```python
from build123d import *

# Parameters (mm, degrees)
F0_W         = 22.86
F0_H         = 48.26
F1_DEPTH     = 50.8
F2_W         = 15.24
F2_H         = 6.35
F3_DEPTH     = 41.91
F4_T1_DEPTH  = 3.81
F4_T3_DEPTH  = 3.81
F4_T8_DEPTH  = 56.8427535009
F4_T14_DEPTH = 56.8427535009
F4_T20_DEPTH = 56.8427535009
F4_T26_DEPTH = 56.8427535009
F5_R         = 7.61999
F6_DEPTH     = 2.54
F7_R         = 3.81
F8_R         = 2.54
F9_DEPTH     = 25.4


# Not quite as in the source:
# - a fillet or chamfer that OpenCascade refuses, or shapes differently, is made with other operations: its cross-section is extruded or revolved along the edge and cut away or added
# - a fillet or chamfer is up to 0.001 mm smaller than in the source, because OpenCascade refuses the exact size


with BuildPart() as f1:
    # F0 (on Top) → F1 (new body)
    with BuildSketch(Plane.XY):
        Rectangle(F0_W, F0_H)
    extrude(amount=F1_DEPTH)

    # F2 (on face) → F3 (cut)
    with BuildSketch(Plane.XY.offset(50.8)):
        Polygon((11.43, 24.13), (-11.43, 24.13), (-11.43, 12.7), (-7.62, 12.7), (7.62, 12.7), (11.43, 12.7), align=None)
        with Locations((0, 9.525)):
            Rectangle(F2_W, F2_H)
        Polygon((-11.43, -12.7), (-11.43, -24.13), (11.43, -24.13), (11.43, -12.7), (7.62, -12.7), (-7.62, -12.7), align=None)
        with Locations((0, -9.525)):
            Rectangle(F2_W, F2_H)
    extrude(amount=-F3_DEPTH, mode=Mode.SUBTRACT)

    # F4: fillet of radius 25.4 on 4 edges, made by hand

    # F4_s2 → F4_t1 (join)
    with BuildSketch(Plane.YZ.offset(-11.43)):
        with BuildLine():
            ThreePointArc((-24.1299175004, 8.889874725), (-15.7392117545, 18.0547879388), (-12.69985, 30.1031013998))
            Line((-12.69985, 30.1031013998), (-12.19185, 30.1031013998))
            ThreePointArc((-12.19185, 30.1031013998), (-12.192, 19.4965506999), (-12.192, 8.89))
            Line((-12.192, 8.89), (-12.7, 8.382))
            ThreePointArc((-12.7, 8.382), (-18.4149587502, 8.382), (-23.8505188504, 8.4656101915))
            Line((-23.8505188504, 8.4656101915), (-24.1299175004, 8.889874725))
        make_face()
        with BuildLine():
            ThreePointArc((24.1299175004, 8.889874725), (15.7392117545, 18.0547879388), (12.69985, 30.1031013998))
            Line((12.69985, 30.1031013998), (12.19185, 30.1031013998))
            ThreePointArc((12.19185, 30.1031013998), (12.192, 19.4965506999), (12.192, 8.89))
            Line((12.192, 8.89), (12.7, 8.382))
            ThreePointArc((12.7, 8.382), (18.4149587502, 8.382), (23.8505188504, 8.4656101915))
            Line((23.8505188504, 8.4656101915), (24.1299175004, 8.889874725))
        make_face()
    extrude(amount=F4_T1_DEPTH)

    # F4_s4 → F4_t3 (join)
    with BuildSketch(Plane.YZ.offset(7.62)):
        with BuildLine():
            ThreePointArc((-24.1299175004, 8.889874725), (-15.7392117545, 18.0547879388), (-12.69985, 30.1031013998))
            Line((-12.69985, 30.1031013998), (-12.19185, 30.1031013998))
            ThreePointArc((-12.19185, 30.1031013998), (-12.192, 19.4965506999), (-12.192, 8.89))
            Line((-12.192, 8.89), (-12.7, 8.382))
            ThreePointArc((-12.7, 8.382), (-18.4149587502, 8.382), (-23.8505188504, 8.4656101915))
            Line((-23.8505188504, 8.4656101915), (-24.1299175004, 8.889874725))
        make_face()
        with BuildLine():
            ThreePointArc((24.1299175004, 8.889874725), (15.7392117545, 18.0547879388), (12.69985, 30.1031013998))
            Line((12.69985, 30.1031013998), (12.19185, 30.1031013998))
            ThreePointArc((12.19185, 30.1031013998), (12.192, 19.4965506999), (12.192, 8.89))
            Line((12.192, 8.89), (12.7, 8.382))
            ThreePointArc((12.7, 8.382), (18.4149587502, 8.382), (23.8505188504, 8.4656101915))
            Line((23.8505188504, 8.4656101915), (24.1299175004, 8.889874725))
        make_face()
    extrude(amount=F4_T3_DEPTH)


with BuildPart() as f4_tool6:
    # F4_s7 → F4_t8 (new body)
    with BuildSketch(Plane.YZ.offset(45.4127535009)):
        with BuildLine():
            ThreePointArc((-24.1299175004, 8.889874725), (-15.7392117545, 18.0547879388), (-12.69985, 30.1031013998))
            Line((-12.69985, 30.1031013998), (-12.19185, 30.1031013998))
            ThreePointArc((-12.19185, 30.1031013998), (-12.192, 19.4965506999), (-12.192, 8.89))
            Line((-12.192, 8.89), (-12.7, 8.382))
            ThreePointArc((-12.7, 8.382), (-18.4149587502, 8.382), (-23.8505188504, 8.4656101915))
            Line((-23.8505188504, 8.4656101915), (-24.1299175004, 8.889874725))
        make_face()
    extrude(amount=-F4_T8_DEPTH)

    split(bisect_by=Plane.YZ.offset(11.43), keep=Keep.BOTTOM)

    split(bisect_by=Plane.YZ.offset(7.62), keep=Keep.TOP)


with BuildPart() as f1_1:
    add(f1.part)

    # F4_t5: union F4_tool6
    add(f4_tool6.part)


with BuildPart() as f4_tool12:
    # F4_s13 → F4_t14 (new body)
    with BuildSketch(Plane.YZ.offset(11.43)):
        with BuildLine():
            ThreePointArc((-24.1299175004, 8.889874725), (-15.7392117545, 18.0547879388), (-12.69985, 30.1031013998))
            Line((-12.69985, 30.1031013998), (-12.19185, 30.1031013998))
            ThreePointArc((-12.19185, 30.1031013998), (-12.192, 19.4965506999), (-12.192, 8.89))
            Line((-12.192, 8.89), (-12.7, 8.382))
            ThreePointArc((-12.7, 8.382), (-18.4149587502, 8.382), (-23.8505188504, 8.4656101915))
            Line((-23.8505188504, 8.4656101915), (-24.1299175004, 8.889874725))
        make_face()
    extrude(amount=-F4_T14_DEPTH)

    split(bisect_by=Plane.YZ.offset(-11.43), keep=Keep.TOP)

    split(bisect_by=Plane.YZ.offset(-7.62), keep=Keep.BOTTOM)


with BuildPart() as f1_2:
    add(f1_1.part)

    # F4_t11: union F4_tool12
    add(f4_tool12.part)


with BuildPart() as f4_tool18:
    # F4_s19 → F4_t20 (new body)
    with BuildSketch(Plane.YZ.offset(-11.43)):
        with BuildLine():
            ThreePointArc((24.1299175004, 8.889874725), (15.7392117545, 18.0547879388), (12.69985, 30.1031013998))
            Line((12.69985, 30.1031013998), (12.19185, 30.1031013998))
            ThreePointArc((12.19185, 30.1031013998), (12.192, 19.4965506999), (12.192, 8.89))
            Line((12.192, 8.89), (12.7, 8.382))
            ThreePointArc((12.7, 8.382), (18.4149587502, 8.382), (23.8505188504, 8.4656101915))
            Line((23.8505188504, 8.4656101915), (24.1299175004, 8.889874725))
        make_face()
    extrude(amount=F4_T20_DEPTH)

    split(bisect_by=Plane.YZ.offset(11.43), keep=Keep.BOTTOM)

    split(bisect_by=Plane.YZ.offset(7.62), keep=Keep.TOP)


with BuildPart() as f1_3:
    add(f1_2.part)

    # F4_t17: union F4_tool18
    add(f4_tool18.part)


with BuildPart() as f4_tool24:
    # F4_s25 → F4_t26 (new body)
    with BuildSketch(Plane.YZ.offset(-45.4127535009)):
        with BuildLine():
            ThreePointArc((24.1299175004, 8.889874725), (15.7392117545, 18.0547879388), (12.69985, 30.1031013998))
            Line((12.69985, 30.1031013998), (12.19185, 30.1031013998))
            ThreePointArc((12.19185, 30.1031013998), (12.192, 19.4965506999), (12.192, 8.89))
            Line((12.192, 8.89), (12.7, 8.382))
            ThreePointArc((12.7, 8.382), (18.4149587502, 8.382), (23.8505188504, 8.4656101915))
            Line((23.8505188504, 8.4656101915), (24.1299175004, 8.889874725))
        make_face()
    extrude(amount=F4_T26_DEPTH)

    split(bisect_by=Plane.YZ.offset(-11.43), keep=Keep.TOP)

    split(bisect_by=Plane.YZ.offset(-7.62), keep=Keep.BOTTOM)


with BuildPart() as f1_4:
    add(f1_3.part)

    # F4_t23: union F4_tool24
    add(f4_tool24.part)

    # F5 (radius 7.62 in the source; OpenCascade refuses exactly that, so slightly less here)
    f5_edges = [f1_4.edges().sort_by_distance(p)[0] for p in [
        (7.62, 6.35, 29.845),
        (-7.62, 6.35, 29.845),
        (7.62, -6.35, 29.845),
        (-7.62, -6.35, 29.845),
    ]]
    fillet(f5_edges, radius=F5_R)

    # F6 (cut): faces of the model
    f6_faces = [f1_4.faces().sort_by_distance(p)[0] for p in [
        (0, 15.9681179393, 8.89),
        (0, -15.9681179393, 8.89),
    ]]
    extrude(f6_faces, amount=-F6_DEPTH, mode=Mode.SUBTRACT)

    # F7
    f7_edges = [f1_4.edges().sort_by_distance(p)[0] for p in [
        (9.525, 24.129727, 8.89),
        (9.525, -24.129727, 8.89),
        (-9.525, 24.129727, 8.89),
        (-9.525, -24.129727, 8.89),
    ]]
    fillet(f7_edges, radius=F7_R)

    # F8 (on face) → F9 (cut)
    with BuildSketch(Plane.XY.offset(6.35)):
        with Locations((0, -19.05)):
            Circle(F8_R)
        with Locations((0, 19.05)):
            Circle(F8_R)
    extrude(amount=-F9_DEPTH, mode=Mode.SUBTRACT)


solid = f1_4.part
```
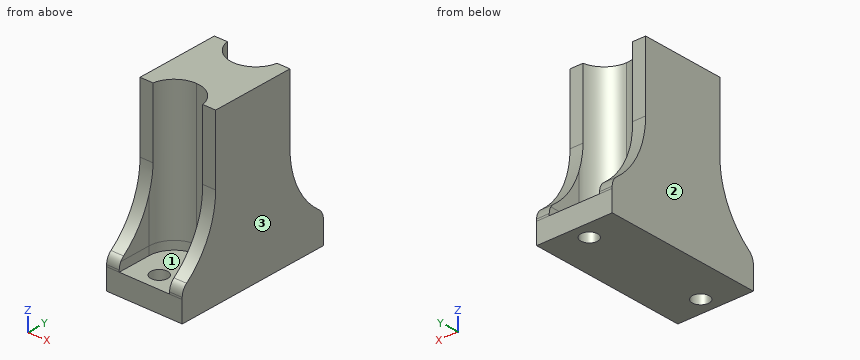
Geometry check sheet. Reference: the model listing, model coordinates, mm. Face numbers are marked on the shaded views. Give positions to 0.01 mm unless a question says otherwise; leave off trailing zeros. Order: outer loops, then holes, each group sorted by start corner. A loop starts at its lowest first (then second) coordinate and runs counter-clockwise, first axis right, second up. Notation, with made-up numbers: (22, -4) -> (30, -4) arc R25 cw to (30, 11) -> close; hole circle Ø8 at (53.5, -2.5). An arc over 180 degrees is marked (long way). Write each question's results on one line, items separated by ' | '. Start each with the question number.
(1) Sectioned sample at D-D (y = -20). Enter the section's corners in (x, z).
(2) Sectioned sample at B-B (y = 21). Enter the section's corners in (x, z), plus the area to 3 significant figures.
(3) Sectioned sample at A-A (x = 1.25). Enter the section's corners in (y, z).
(4) Scan lines: line 1 (Y direction, x = 0, z = 2.5); line 2 (Y direction, x = 2.25, z = 4); line 3 (X direction, y = 19, z = 4). Record each from-to range of solid material in increasing order.
(5) Gauge pin test, flat ends, axial feed: P1, Ø4, axis at x = 0, y = 19.05, coming from the +Z side; P2, Ø1.2, axis at x = -10, z = 40.5, coming from the -Y side; P3, Ø5, axis at x = -3.5, z = 29.5, coming from the +Y side. Record the tip position at first contact, or that the pin passes through.
(6) Mould release check, pull along X, two halves, no side actions. Record for the marked faces 1, 2 and 3: pulls with the +X half, pulls with the -X half, needs draft (parallel to the pull), parting line crosses it, or undercut.
Answer below:
1) outline: (-11.43, 0) -> (-2.36, 0) -> (-2.36, 6.35) -> (-7.62, 6.35) -> (-7.62, 12.28) -> (-11.43, 12.28) -> close; (2.36, 0) -> (11.43, 0) -> (11.43, 12.28) -> (7.62, 12.28) -> (7.62, 6.35) -> (2.36, 6.35) -> close
2) outline: (-11.43, 0) -> (-1.63, 0) -> (-1.63, 6.35) -> (-7.62, 6.35) -> (-7.62, 11.32) -> (-11.43, 11.32) -> close; (1.63, 0) -> (11.43, 0) -> (11.43, 11.32) -> (7.62, 11.32) -> (7.62, 6.35) -> (1.63, 6.35) -> close | area: 162 mm2
3) outline: (-24.13, 0) -> (-21.26, 0) -> (-21.26, 6.35) -> (-24.13, 6.35) -> close; (-16.84, 0) -> (16.84, 0) -> (16.84, 6.35) -> (6.45, 6.35) -> (6.45, 50.8) -> (-6.45, 50.8) -> (-6.45, 6.35) -> (-16.84, 6.35) -> close; (21.26, 0) -> (24.13, 0) -> (24.13, 6.35) -> (21.26, 6.35) -> close
4) line 1: -24.13 to -21.59, -16.51 to 16.51, 21.59 to 24.13 | line 2: -24.13 to -20.23, -17.87 to 17.87, 20.23 to 24.13 | line 3: -11.43 to -2.54, 2.54 to 11.43
5) P1: through | P2: y = -12.7 | P3: y = 9.27
6) face 1: undercut | face 2: pulls with the -X half | face 3: pulls with the +X half
